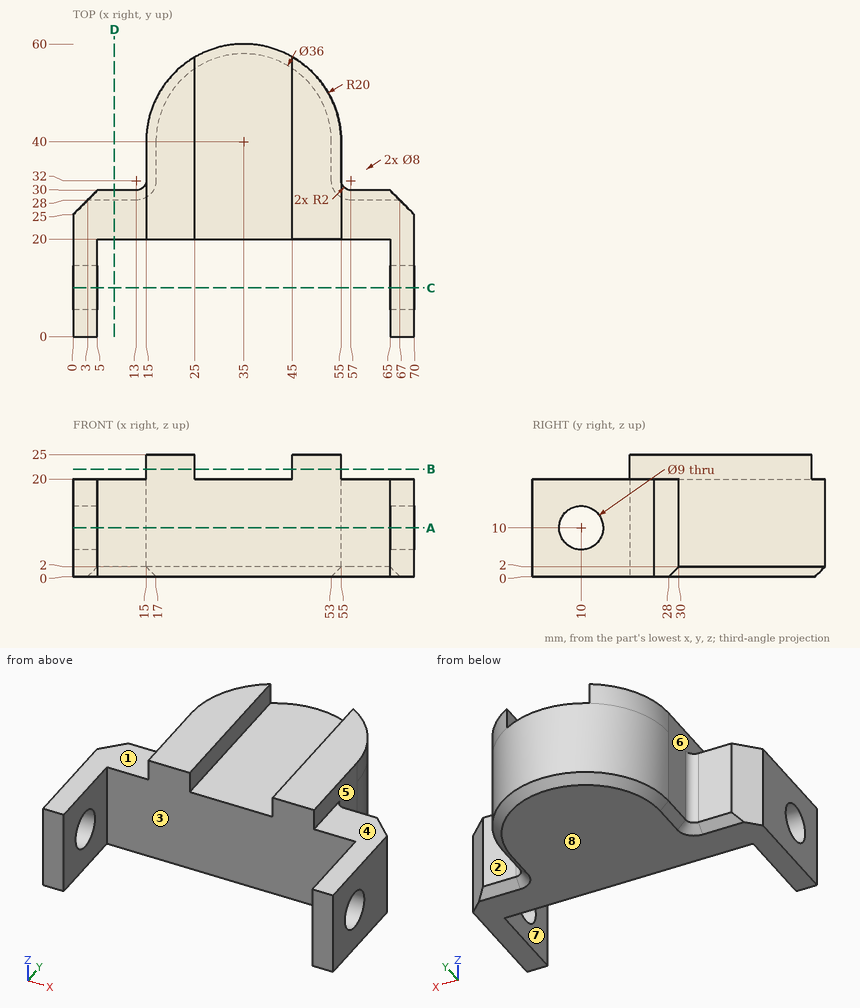
Here's the drawing with two shaded views (mm, measured from the low corner). I have some questions. A direction names the side the tool comes from. Coordinates: 2 decimals unless noted, no trailing zeros. Loops run counter-clockwise (first coordinate to the right, second up) from the corner with the lowest first, then second, coordinate; pieces in that order, holes last.
Item 1: Suppose I cut it at C-C (y = 10). Please give me the cut outline in (x, z), then the cut area to 3 significant figures.
Answers below:
outline: (0, 0) - (5, 0) - (5, 5.5) - (0, 5.5) - close; (0, 14.5) - (5, 14.5) - (5, 20) - (0, 20) - close; (65, 0) - (70, 0) - (70, 5.5) - (65, 5.5) - close; (65, 14.5) - (70, 14.5) - (70, 20) - (65, 20) - close
area: 110 mm2
Item 2: Suppose I cut it at A-A (z = 10). Please give me the cut outline in (x, y), then the cut area to 3 significant figures.
Answers below:
outline: (0, 0) - (5, 0) - (5, 5.5) - (0, 5.5) - close; (0, 14.5) - (5, 14.5) - (5, 20) - (65, 20) - (65, 14.5) - (70, 14.5) - (70, 25) - (65, 30) - (57, 30) arc R2 cw to (55, 32) - (55, 40) arc R20 ccw to (15, 40) - (15, 32) arc R2 cw to (13, 30) - (5, 30) - (0, 25) - close; (65, 0) - (70, 0) - (70, 5.5) - (65, 5.5) - close
area: 1,820 mm2
Item 3: If we mould it in two halves opening along X, with no side actions, what happens to the marked faces 6, 7 and 8? For each: released by +X, released by -X, zero draft, split by the parting line, or undercut.
Answers below:
face 6: released by -X
face 7: undercut
face 8: zero draft
Item 4: I'm going to push flat-ended pins straight in: pin 1 (1.5 mm diameter, centred on y = 29.5, z = 22.5, fed in from +X); pin 2 (5 mm diameter, centred on x = 54.5, z = 21.5, fed in from -Y); pin 3 (10 mm diameter, centred on y = 34.5, z = 5, fed in from -X); pin 4 (4.5 mm diameter, centred on x = 61, y = 13.5, fed in from +Z). Where does each tip first touch, or does it pass through?
Answers below:
pin 1: stops at x = 55
pin 2: stops at y = 20
pin 3: stops at x = 4.5
pin 4: passes through
Item 5: Suppose I cut it at B-B (z = 22). Please give me the cut outline in (x, y).
Answers below:
outline: (15, 20) - (25, 20) - (25, 57.32) arc R20 ccw to (15, 40) - close; (45, 20) - (55, 20) - (55, 40) arc R20 ccw to (45, 57.32) - close
Item 6: Please list where these lines run through material, in increasing order: L1, parallel to X at y = 11.5, z = 4.75; L2, parallel to Y at x = 9, z = 7.75; L3, parallel to Y at x = 3.35, z = 10.
Answers below:
L1: x = 0 to 5, 65 to 70
L2: y = 20 to 30
L3: y = 0 to 5.5, 14.5 to 28.35
Item 7: Suppose I cut it at D-D (x = 8.5). Please give me the cut outline in (y, z).
Answers below:
outline: (20, 0) - (28, 0) - (30, 2) - (30, 20) - (20, 20) - close
Item 8: Which directions (+Z, -Z, +X, -X, +Y, -Y) give clear straight access to the entire face, cutting with the end or side of a thin tool? Please do the marked faces 1, 2, 3, 4 and 5.
Answers below:
face 1: +Z, -X, +Y, -Y
face 2: +Z, -Z, +X, +Y
face 3: +Z, -Z, -Y
face 4: +Z, +X, +Y, -Y
face 5: +Z, +X, +Y
